from build123d import *

# Parameters (mm, degrees)
EXTRUDE_1_DEPTH             = 10
HOLE_WIZARD_M41_D           = 4.5
HOLE_WIZARD_M41_CBORE_D     = 8
HOLE_WIZARD_M41_CBORE_DEPTH = 4


with BuildPart() as part:
    # Эскиз1 → Бобышка-Вытянуть1 (new body)
    with BuildSketch(Plane.XY):
        with BuildLine():
            ThreePointArc((0, -5), (1.97749323, -4.592332798), (3.632522807, -3.43580821))
            add(Edge.make_bspline(
                [(15.044141894, -1.499350357), (10.394641273, -1.355433826), (5.459325404, -1.902106002), (3.632522807, -3.43580821)],
                knots=[0, 0, 0, 0, 1, 1, 1, 1], degree=3))
            ThreePointArc((15.044141894, -1.499350357), (16.456610687, -0.358169384), (15.734424867, 1.307906768))
            add(Edge.make_bspline(
                [(15.734424867, 1.307906768), (10.086793818, 4.339667199), (3.284920128, 5.036214544), (0, 5)],
                knots=[0, 0, 0, 0, 1, 1, 1, 1], degree=3))
            ThreePointArc((0, 5), (-1.97749323, 4.592332798), (-3.632522807, 3.43580821))
            add(Edge.make_bspline(
                [(-15.044141894, 1.499350357), (-10.394641273, 1.355433826), (-5.459325404, 1.902106002), (-3.632522807, 3.43580821)],
                knots=[0, 0, 0, 0, 1, 1, 1, 1], degree=3))
            ThreePointArc((-15.044141894, 1.499350357), (-16.456610687, 0.358169384), (-15.734424867, -1.307906768))
            add(Edge.make_bspline(
                [(-15.734424867, -1.307906768), (-10.086793818, -4.339667199), (-3.284920128, -5.036214544), (0, -5)],
                knots=[0, 0, 0, 0, 1, 1, 1, 1], degree=3))
        make_face()
    extrude(amount=EXTRUDE_1_DEPTH)

    # Цековка для винта с внутренним шестигранником M41 (through all)
    with Locations(Plane.XY.offset(10)):
        with Locations((0, 0)):
            CounterBoreHole(HOLE_WIZARD_M41_D / 2, HOLE_WIZARD_M41_CBORE_D / 2, HOLE_WIZARD_M41_CBORE_DEPTH)


solid = part.part
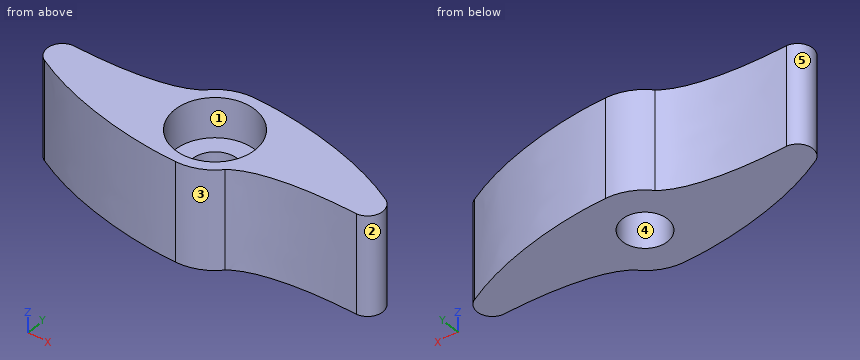
Work out the finished part from the listing and answer in its coordinate system (mm). Face numbers are marked on the shaded views. A direction names the side the tool comes from. Round coordinates to 2 decimals unless told otherwise and drop trailing zeros. Write each loop counter-clockwise with the first axis right and the second up, starting at its lowest first coordinate (ties: lowest second). Pieces come first, ordered by that corner, then holes. Notation, with made-up numbers: (-34.75, -33.75) - (11.25, -33.75) arc R17 ccw to (11.25, -9.75) - close; hole circle Ø4 at (28, 16). An arc over 180 degrees is marked (long way). Answer in a Markdown table with one row per item. Add a question column.
1. A cutting plane is placed at A-A, the plane y = 0. Determine the outline of the cut face in (x, z).
2. Find the intervals of material crossed by line 1 along Y through (x, z) = (0, 8.55); line 2 along Y through (x, z) = (0, 2.05); line 3 along X through (y, z) = (-0.75, 3), in increasing order. Write a range as from..to.
3. For the marked faces 1 and 2, determine the directions among +Z, -Z, +X, -X, +Y, -Y from which every point of the face is accessible in a straight line to the end or side of a thin tool.
4. Given pin 1 (3 mm diameter, centred on x = 13, z = 5.5, fed in from +Y); pin 2 (1.5 mm diameter, centred on x = -11, z = 6.5, fed in from +Y); pin 3 (4 mm diameter, centred on y = 3.5, z = 7, fed in from +X); pin 4 (3.5 mm diameter, centred on x = 0, y = 0, fed in from +Z), each flat-ended and moving along its own axis, determine where each tip first touches the part or whether it passes through.
5. The mould has two halves that part along Y. Classify the marked faces 3, 4 and 5: +Y half, -Y half, draft (parallel to the pull), parting line (faces both ways), or undercut.
Worked out:
| question | item | result |
|---|---|---|
| 1 | outline | (-16.5, 0) - (-2.25, 0) - (-2.25, 6) - (-4, 6) - (-4, 10) - (-16.5, 10) - close; (2.25, 0) - (16.5, 0) - (16.5, 10) - (4, 10) - (4, 6) - (2.25, 6) - close |
| 2 | line 1 | -5..-4, 4..5 |
| 2 | line 2 | -5..-2.25, 2.25..5 |
| 2 | line 3 | -16.3..-2.12, 2.12..16.3 |
| 3 | face 1 | +Z |
| 3 | face 2 | +Z, -Z, +X |
| 4 | pin 1 | y = 3.12 |
| 4 | pin 2 | y = 1.61 |
| 4 | pin 3 | x = 15.37 |
| 4 | pin 4 | through |
| 5 | face 3 | -Y half |
| 5 | face 4 | undercut |
| 5 | face 5 | parting line |
